Source: CAD feature listing. Evaluate the final solid. Frame: model axes, mm. A direction names the side the tool comes from. Coordinates: 2 decimals unless noted, no trailing zeros. Write each loop counter-clockwise with the first axis right and the second up, starting at its lowest first coordinate (ties: lowest second). Pieces come first, ordered by that corner, then holes. Notation, with made-up numbers: (1, 27) -> (55, 27) arc R27 ccw to (55, 49) -> close; hole circle Ø5 at (60, 71). An arc over 180 degrees is marked (long way). Write item = value, one per line.
from build123d import *

# Parameters (mm, degrees)
SKETCH1_W               = 50
SKETCH1_H               = 150
BOSS_EXTRUDE1_DEPTH     = 420
CUT_EXTRUDE1_DEPTH      = 400
CUT_EXTRUDE1_DEPTH_BACK = 400
SKETCH2_R               = 20
SKETCH3_R               = 50
BOSS_EXTRUDE2_DEPTH     = 10


with BuildPart() as part:
    # Sketch1 → Boss-Extrude1 (new body)
    with BuildSketch(Plane.XY):
        Rectangle(SKETCH1_W, SKETCH1_H)
    extrude(amount=BOSS_EXTRUDE1_DEPTH)

    # Sketch2 → Cut-Extrude1 (cut, two sides: drawn at the far end of the back side and taken through both)
    with BuildSketch(Plane(origin=(25, 0, 0), x_dir=(0, 0, -1), z_dir=(1, 0, 0)).offset(-CUT_EXTRUDE1_DEPTH_BACK)):
        with Locations(Location((-320, 0, 0), (0, 0, 180))):
            Circle(SKETCH2_R)
    extrude(amount=CUT_EXTRUDE1_DEPTH + CUT_EXTRUDE1_DEPTH_BACK, mode=Mode.SUBTRACT)

    # Sketch3 → Boss-Extrude2 (add)
    with BuildSketch(Plane(origin=(25, 0, 0), x_dir=(0, 0, -1), z_dir=(1, 0, 0))):
        with Locations(Location((-100, 0, 0), (0, 0, 180))):
            Circle(SKETCH3_R)
    extrude(amount=BOSS_EXTRUDE2_DEPTH)


solid = part.part
1) First-contact query: pin 1 Ø1 at (y, z) = (32, 317.5) entering from +X. Flat tip, straight axial feed; report the tip coordinate or a pass-through.
Answer block:
pin_1 = 25
2) Material intervals for probe 1 along Y at (x, z) = (2, 320); probe 2 along X at (y, z) = (56.5, 147); probe 3 along Y at (x, z) = (13, 318), sorted ascending. Write a range as [from, to].
Answer block:
probe_1 = [-75, -20], [20, 75]
probe_2 = [-25, 25]
probe_3 = [-75, -19.9], [19.9, 75]
3) Pull-direction query (Z, two-part tool) for faces 1 (the flat face through (35, -1, 99)), 2 (the flat face through (0, 1, 420)), 3 (the flat face through (0, 1, 0)), 4 (the cylindrical face through (-0.35, 7.66, 338.475)); classes: +Z half, -Z half, draft (parallel to the pull), parting line (faces both ways), or undercut.
Answer block:
face_1 = draft
face_2 = +Z half
face_3 = -Z half
face_4 = undercut
4) Cut plane A-A, the plane y = 0. Output: boundary loops of the cut face in (x, z).
Answer block:
outline = (-25, 0) -> (25, 0) -> (25, 50) -> (35, 50) -> (35, 150) -> (25, 150) -> (25, 300) -> (-25, 300) -> close; (-25, 340) -> (25, 340) -> (25, 420) -> (-25, 420) -> close
5) Reachability of faces 5 (the cylindrical face through (29.93, -2.2, 50.05)), 6 (the flat face through (0, -75, 207)) from +Z, -Z, +X, -X, +Y, -Y: full face, straight path, thin tool, end or side. Return the list, or none.
Answer block:
face_5 = +X
face_6 = +Z, -Z, +X, -X, -Y
6) Cut plane B-B, the plane z = 320. Output: boundary loops of the cut face in (x, y).
Answer block:
outline = (-25, -75) -> (25, -75) -> (25, -20) -> (-25, -20) -> close; (-25, 20) -> (25, 20) -> (25, 75) -> (-25, 75) -> close
7) Cut plane D-D, the plane x = 7. Output: boundary loops of the cut face in (y, z).
Answer block:
outline = (-75, 0) -> (75, 0) -> (75, 420) -> (-75, 420) -> close; hole circle Ø40 at (0, 320)
8) Cut plane C-C, the plane z = 100. Output: boundary loops of the cut face in (x, y).
Answer block:
outline = (-25, -75) -> (25, -75) -> (25, -50) -> (35, -50) -> (35, 50) -> (25, 50) -> (25, 75) -> (-25, 75) -> close
